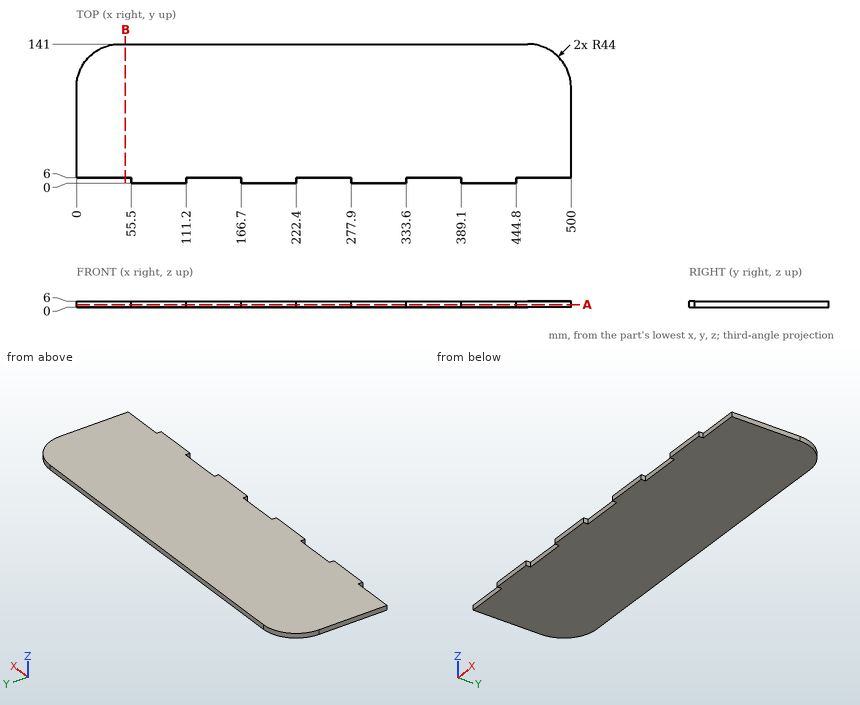
Job drawing, mm, ordinate dimensions from the low corner. One solid piece. Give positions to 0.01 mm unless a question says otherwise; leave off trailing zeros. Loops run counter-clockwise (first coordinate to the right, second up) from the corner with the lowest first, then second, coordinate; pieces in that order, holes last. Notation, with made-up numbers: (-19.5, 0.5) -> (-1.5, 0.5) arc R12 cw to (-1.5, 9.5) -> close; hole circle Ø11 at (20.25, 36). An arc over 180 degrees is marked (long way). Use a Markdown table: item, result. Add a question column.
(1) Slice it at A-A on z = 2.8. List the corners of the cut face in (x, y).
(2) Drop flat-ended pins along their axis: pin 1 Ø1.8 at (x, z) = (364, 3) entering from -Y; pin 2 Ø1.8 at (y, z) = (3.5, 2.5) entering from +X; pin 3 Ø1.8 at (y, z) = (3.5, 4.5) entering from -X. Give the stop position or say it passes through.
(3) Slice it at B-B on x = 49.5. List the corners of the cut face in (y, z), and give its area (3 significant figures).
(4) Wall check: line 1 along Y through (x, z) = (139, 3.4); line 2 along X through (y, z) = (118, 3.5); line 3 along X through (y, z) = (101, 3.6). Give the ranges that are in metal, low to high.
Filled sheet:
| question | item | result |
|---|---|---|
| 1 | outline | (0, 6) -> (55.5, 6) -> (55.5, 0) -> (111.2, 0) -> (111.2, 6) -> (166.7, 6) -> (166.7, 0) -> (222.4, 0) -> (222.4, 6) -> (277.9, 6) -> (277.9, 0) -> (333.6, 0) -> (333.6, 6) -> (389.1, 6) -> (389.1, 0) -> (444.8, 0) -> (444.8, 6) -> (500, 6) -> (500, 97) arc R44 ccw to (456, 141) -> (44, 141) arc R44 ccw to (0, 97) -> close |
| 2 | pin 1 | y = 6 |
| 2 | pin 2 | x = 444.8 |
| 2 | pin 3 | x = 55.5 |
| 3 | outline | (6, 0) -> (141, 0) -> (141, 6) -> (6, 6) -> close |
| 3 | area | 810 mm2 |
| 4 | line 1 | 6 to 141 |
| 4 | line 2 | 5.33 to 494.67 |
| 4 | line 3 | 0.18 to 499.82 |
